Source: CAD feature listing. Evaluate the final solid. Frame: model axes, mm. Face numbers are marked on the shaded views. Round coordinates to 2 decimals unless told otherwise and drop trailing zeros. Loops run counter-clockwise (first coordinate to the right, second up) from the corner with the lowest first, then second, coordinate; pieces in that order, holes last.
Item 1: Section query B-B on z = -8. Give the number of separate pieces and of enclosed holes in the cut face, then the cut area to 3 significant figures.
Item 2: First-contact query: P1, Ø1, axis at y = -3, z = 8.5, coming from the +X side; P2, Ø3, axis at y = -3, z = 11, coming from the -X side; P3, Ø1.5, axis at y = -6, z = -6, coming from the +X side; P4, Ø6, axis at x = 21.5, z = 3.5, coming from the +Y side. Flat tips, straight axial feed; report the tip coordinate or a pass-through.
Item 3: Section query A-A on x = 0. Return loops of the section in (y, z), then the cut area to 3 significant figures.
Item 4: Pull-direction query (X, two-part tool) for the marked faces 1 and 2; classes: released by +X, released by -X, zero draft, split by the parting line, or undercut.
Item 5: Ray query, L1, parallel to X at y = -5.5, z = 3; L2, parallel to X at y = -2.25, z = -8.5; L3, parallel to X at y = -1.75, z = 14. Return the intervals inside material, ascending.
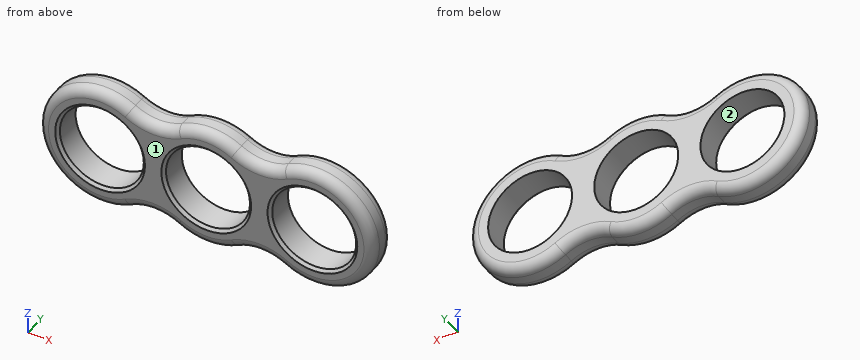
```python
from build123d import *

# Parameters (mm, degrees)
F0_R     = 11.049
F1_DEPTH = 7.62
F2_R     = 2.54
F3_SIZE  = 0.762


with BuildPart() as f1:
    # F0 (on Front) → F1 (new body)
    with BuildSketch(Plane.XZ):
        with BuildLine():
            ThreePointArc((-20.148096, -14.074648), (-13.991215, -12.494351), (-7.839726, -14.095508))
            ThreePointArc((-7.839726, -14.095508), (0, -16.129), (7.839726, -14.095508))
            ThreePointArc((7.839726, -14.095508), (13.991215, -12.494351), (20.148096, -14.074648))
            ThreePointArc((20.148096, -14.074648), (44.068977, 0.074687), (20.100274, 14.142859))
            ThreePointArc((20.100274, 14.142859), (13.948785, 12.541703), (7.791904, 14.122))
            ThreePointArc((7.791904, 14.122), (0, 16.129), (-7.791904, 14.122))
            ThreePointArc((-7.791904, 14.122), (-13.948785, 12.541703), (-20.100274, 14.142859))
            ThreePointArc((-20.100274, 14.142859), (-44.068977, 0.074687), (-20.148096, -14.074648))
        make_face()
        Circle(F0_R, mode=Mode.SUBTRACT)
        with Locations((-27.94, 0.047352)):
            Circle(F0_R, mode=Mode.SUBTRACT)
        with Locations((27.94, 0.047352)):
            Circle(F0_R, mode=Mode.SUBTRACT)
    extrude(amount=F1_DEPTH)

    # F2
    f2_edges = [f1.edges().sort_by_distance(p)[0] for p in [
        (44.068977, -7.62, 0.074687),
        (44.068977, 0, 0.074687),
    ]]
    fillet(f2_edges, radius=F2_R)

    # F3
    f3_edges = [f1.edges().sort_by_distance(p)[0] for p in [
        (-38.989, -7.62, 0.047352),
        (-11.049, -7.62, 0),
        (16.891, -7.62, 0.047352),
    ]]
    chamfer(f3_edges, length=F3_SIZE)


solid = f1.part
```
Data:
1. separate pieces: 4
1. enclosed holes: 0
1. area: 283 mm2
2. P1: stops at x = 41.97
2. P2: stops at x = -41.01
2. P3: stops at x = 43.08
2. P4: passes through
3. outline: (-7.62, -13.59) arc R2.54 ccw to (-5.08, -16.13) - (-2.54, -16.13) arc R2.54 ccw to (0, -13.59) - (0, -11.05) - (-6.86, -11.05) - (-7.62, -11.81) - close; (-7.62, 11.81) - (-6.86, 11.05) - (0, 11.05) - (0, 13.59) arc R2.54 ccw to (-2.54, 16.13) - (-5.08, 16.13) arc R2.54 ccw to (-7.62, 13.59) - close
3. area: 71.3 mm2
4. face 1: zero draft
4. face 2: undercut
5. L1: x = -43.76 to -38.59, -17.29 to -10.63, 10.63 to 17.29, 38.59 to 43.76
5. L2: x = -41.6 to -34.94, -20.94 to -7.06, 7.06 to 20.94, 34.94 to 41.6
5. L3: x = -35.78 to -20.1, -7.75 to 7.75, 20.1 to 35.78
